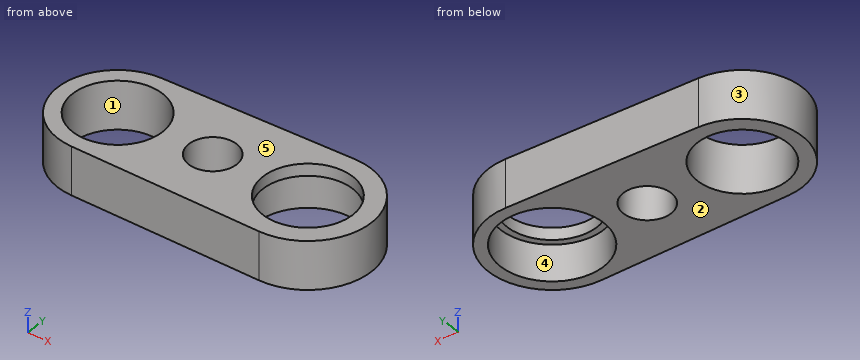
from build123d import *

# Parameters (mm, degrees)
SKETCH_R        = 7.5
SKETCH_R_2      = 4
PAD_DEPTH       = 8
SKETCH001_R     = 8.6
POCKET_DEPTH    = 6
POCKET001_DEPTH = 8.001


with BuildPart() as part:
    # Sketch → Pad (new body)
    with BuildSketch(Plane.XY):
        with BuildLine():
            ThreePointArc((-32.1875, 9.998242), (-42, 0), (-32.1875, -9.998242))
            Line((-32.1875, -9.998242), (-0.19875, -10.598137))
            ThreePointArc((-0.19875, -10.598137), (10.6, 0), (-0.19875, 10.598137))
            Line((-32.1875, 9.998242), (-0.19875, 10.598137))
        make_face()
        with Locations((-32, 0)):
            Circle(SKETCH_R, mode=Mode.SUBTRACT)
        Circle(SKETCH_R, mode=Mode.SUBTRACT)
        with Locations((-16, 0)):
            Circle(SKETCH_R_2, mode=Mode.SUBTRACT)
    extrude(amount=PAD_DEPTH)

    # Sketch001 → Pocket (cut)
    with BuildSketch(Plane(origin=(0, 0, 0), x_dir=(1, 0, 0), z_dir=(0, 0, -1))):
        Circle(SKETCH001_R)
    extrude(amount=-POCKET_DEPTH, mode=Mode.SUBTRACT)

    # Sketch002 → Pocket001 (cut, through all)
    with BuildSketch(Plane(origin=(0, 0, 0), x_dir=(1, 0, 0), z_dir=(0, 0, -1))):
        Polygon((-34.829016, 4.9), (-37.658033, 0), (-34.829016, -4.9), (-29.170984, -4.9), (-26.341967, 0), (-29.170984, 4.9), align=None)
    extrude(amount=-POCKET001_DEPTH, mode=Mode.SUBTRACT)


solid = part.part
Could you check a few things on this model? Use its own coordinates, in mm. Face numbers are marked on the shaded views. A direction names the side the tool comes from. Give positions to 0.01 mm unless a question says otherwise; leave off trailing zeros. Write each loop counter-clockwise with the first axis right and the second up, starting at its lowest first coordinate (ties: lowest second). Pieces come first, ordered by that corner, then holes. Notation, with made-up numbers: (16.25, -30.75) -> (61.25, -30.75) arc R10 cw to (61.25, -14.75) -> close; hole circle Ø8 at (73, 59). An arc over 180 degrees is marked (long way). Answer as CSV lines item,"result". Start each with the question number.
(1) Which directions (+Z, -Z, +X, -X, +Y, -Y) give clear straight access to the entire face, cutting with the end or side of a thin tool? Please do the marked faces 4 and 5.
(2) If we section it at D-D, the plane y = -0.75: Write out the boundary of the cut face in (x, z), and give its area (3 significant figures).
(3) If we mould it in two halves opening along X, with no side actions, what happens to the marked faces 1, 2 and 3? For each: +X half, -X half, draft (parallel to the pull), parting line (faces both ways), or undercut.
(4) Please list where these lines run through material, in increasing order: line 1 (Y direction, x = 0, z = 6.55); line 2 (Y direction, x = -32, z = 4.25); line 3 (X direction, y = 2, z = 2).
(5) If we section it at B-B, the plane z = 0.5: Write out the boundary of the cut face in (x, y), and give its area (3 significant figures).
(6) If we section it at C-C, the plane y = -4.5: Write out the boundary of the cut face in (x, z), and give its area (3 significant figures).
(7) If we section it at A-A, the plane x = -1.5: Write out the boundary of the cut face in (y, z), and give its area (3 significant figures).
(8) I'm going to push flat-ended pins straight in: pin 1 Ø1 at (x, z) = (-4.5, 1.5) entering from +Y; pin 2 Ø1 at (y, z) = (-3, 3.5) entering from -X; pin 3 Ø1.5 at (y, z) = (-5, 3.5) entering from -X. Where does each tip first touch, or does it pass through?
Answer list:
1,face 4,"-Z"
1,face 5,"+Z, +X, -X, +Y, -Y"
2,outline,"(-41.97, 0) -> (-39.46, 0) -> (-39.46, 8) -> (-41.97, 8) -> close; (-24.54, 0) -> (-19.93, 0) -> (-19.93, 8) -> (-24.54, 8) -> close; (-12.07, 0) -> (-8.57, 0) -> (-8.57, 6) -> (-7.46, 6) -> (-7.46, 8) -> (-12.07, 8) -> close; (7.46, 6) -> (8.57, 6) -> (8.57, 0) -> (10.57, 0) -> (10.57, 8) -> (7.46, 8) -> close"
2,area,"105 mm^2"
3,face 1,"undercut"
3,face 2,"draft"
3,face 3,"-X half"
4,line 1,"-10.6 to -7.5, 7.5 to 10.6"
4,line 2,"-10 to -7.5, 7.5 to 10"
4,line 3,"-41.8 to -39.23, -24.77 to -19.46, -12.54 to -8.36, 8.36 to 10.41"
5,outline,"(-32.19, -10) -> (-0.2, -10.6) arc R10.6 ccw (long way) to (-0.2, 10.6) -> (-32.19, 10) arc R10 ccw to start; hole circle Ø15 at (-32, 0); hole circle Ø8 at (-16, 0); hole circle Ø17.2 at (0, 0)"
5,area,"534 mm^2"
6,outline,"(-40.93, 0) -> (-38, 0) -> (-38, 8) -> (-40.93, 8) -> close; (-26, 0) -> (-7.33, 0) -> (-7.33, 6) -> (-6, 6) -> (-6, 8) -> (-26, 8) -> close; (6, 6) -> (7.33, 6) -> (7.33, 0) -> (9.6, 0) -> (9.6, 8) -> (6, 8) -> close"
6,area,"196 mm^2"
7,outline,"(-10.57, 0) -> (-8.47, 0) -> (-8.47, 6) -> (-7.35, 6) -> (-7.35, 8) -> (-10.57, 8) -> close; (7.35, 6) -> (8.47, 6) -> (8.47, 0) -> (10.57, 0) -> (10.57, 8) -> (7.35, 8) -> close"
7,area,"38.2 mm^2"
8,pin 1,"y = 10.53"
8,pin 2,"x = -41.68"
8,pin 3,"x = -41.05"
